from build123d import *

# Parameters (mm, degrees)
SKETCH2_R          = 3.3655
CUT_EXTRUDE1_DEPTH = 19.05
CIRPATTERN1_COUNT  = 4


with BuildPart() as part:
    # Sketch1 → Revolve1 (revolve)
    with BuildSketch(Plane(origin=(0, 0, 0), x_dir=(0, 0, -1), z_dir=(1, 0, 0)), mode=Mode.PRIVATE) as revolve1_sk:
        Polygon((-1.27, 26.924), (10.6426, 26.924), (10.6426, 12.827), (0, 12.827), (0, 13.97), (-0.635, 14.201121099), (0.205363195, 16.51), (-1.27, 16.51), align=None)
    revolve(revolve1_sk.sketch.rotate(Axis((0, 0, 0), (0, 0, 1)), 90), axis=Axis((0, 0, 0), (0, 0, 1)))

    # Sketch2 → Cut-Extrude1 (cut, symmetric)
    with BuildSketch(Plane.XY):
        with Locations(Location((0, 20.6375, 0), (0, 0, 180))):
            Circle(SKETCH2_R)
    cut_extrude1 = extrude(amount=CUT_EXTRUDE1_DEPTH, both=True, mode=Mode.SUBTRACT)

    # CirPattern1: Cut-Extrude1 ×4 about axis
    cirpattern1_axis = Axis((0, 0, 0), (0, 0, 1))
    for i in range(1, CIRPATTERN1_COUNT):
        add(cut_extrude1.rotate(cirpattern1_axis, i * 360 / CIRPATTERN1_COUNT), mode=Mode.SUBTRACT)


solid = part.part
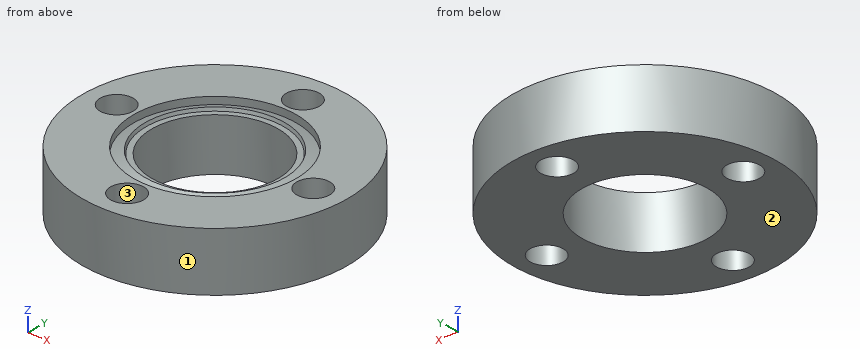
Verification items for the finished model (mm, model axes). Face numbers are marked on the shaded views. Give positions to 0.01 mm unless a question says otherwise; leave off trailing zeros. Write each loop counter-clockwise with the first axis right and the second up, starting at its lowest first coordinate (ties: lowest second). Pieces come first, ordered by that corner, then holes. Notation, with made-up numbers: M 68,58.5 L 99,58.5 A16 ccw 99,69.5 Z; hole C -29.75,86.25 d4. An arc over 180 degrees is marked long. Write item = value, one per line.
(1) Sectioned sample at A-A (y = 0). Record the cut outline in (x, z) (3 decimals), then the cut area to 3 significant figures.
Found:
outline = M -26.924,-10.643 L -24.003,-10.643 L -24.003,1.27 L -26.924,1.27 Z; M -17.272,-10.643 L -12.827,-10.643 L -12.827,0 L -13.97,0 L -14.201,0.635 L -16.51,-0.205 L -16.51,1.27 L -17.272,1.27 Z; M 12.827,-10.643 L 17.272,-10.643 L 17.272,1.27 L 16.51,1.27 L 16.51,-0.205 L 14.201,0.635 L 13.97,0 L 12.827,0 Z; M 24.003,-10.643 L 26.924,-10.643 L 26.924,1.27 L 24.003,1.27 Z
area = 167 mm2
(2) Material ranges on line 1 (Y direction, x = 0, z = -2); line 2 (Y direction, x = -1, z = -9); line 3 (Z direction, x = 8, y = 11), recorded low to high.
Found:
line_1 = -26.92 to -24, -17.27 to -12.83, 12.83 to 17.27, 24 to 26.92
line_2 = -26.91 to -23.85, -17.42 to -12.79, 12.79 to 17.42, 23.85 to 26.91
line_3 = -10.64 to 0
(3) Sectioned sample at C-C (z = -2.25). Record the cut outline in (x, y).
Found:
outline = C 0,0 d53.85; hole C -20.64,0 d6.73; hole C 0,0 d25.65; hole C 0,-20.64 d6.73; hole C 0,20.64 d6.73; hole C 20.64,0 d6.73
(4) Draft check along Y on the marked faces 1, 2 and 3. Enter one of: released by +Y, released by -Y, zero draft, split by the parting line, or undercut.
Found:
face_1 = split by the parting line
face_2 = zero draft
face_3 = undercut
(5) Go/stop test with flat-tipped pins: pin 1 Ø1.5 at (x, z) = (-8, -7) entering from +Y; pin 2 Ø1.5 at (x, z) = (10.5, -2) entering from -Y; pin 3 Ø2 at (x, z) = (12.5, -5) entering from +Y. Record where each tip stops, or that it passes through.
Found:
pin_1 = 25.93
pin_2 = -25.1
pin_3 = 24.34
